Verification items for the finished model (mm, model axes). Face numbers are marked on the shaded views. A direction names the side the tool comes from. Round coordinates to 2 decimals unless told otherwise and drop trailing zeros. Write each loop counter-clockwise with the first axis right and the second up, starting at its lowest first coordinate (ties: lowest second). Pieces come first, ordered by that corner, then holes. Notation, with made-up numbers: M 49,-27.75 L 101,-27.75 A14 ccw 101,-20.75 Z; hole C 0.25,25.25 d8. An arc over 180 degrees is marked long. One line per question, with ' | ' between items.
Autodesk Inventor part; units mm, degrees
ref_plane "YZ Plane" through (0, 0, 0) normal (1, 0, 0) x (0, 1, 0)
ref_plane "XZ Plane" through (0, 0, 0) normal (0, 1, 0) x (-1, 0, 0)
ref_plane "XY Plane" through (0, 0, 0) normal (0, 0, 1) x (1, 0, 0)
sketch "Sketch4" plane through (0, 0, 0) normal (0, 0, 1) x (1, 0, 0)
  line L0 (-1.6, 0) -> (5, 0)
  line L1 (0, 0) -> (-1.6, 0)
  line L2 (0, 2) -> (0, 1.38)
  line L3 (0.4, 0.98) -> (0.4, 0.98)
  line L4 (0.4, 0.98) -> (0.8, 1)
  arc A0 (0, 1.38) -> (0.4, 0.98) centre (0.4, 1.38) ccw
  line L5 (-1.6, 0) -> (-1.6, 1)
  line L6 (0, 2) -> (-0.83, 2)
  arc A1 (-0.83, 2) -> (-1.6, 1) centre (1.2707, -0.414) ccw
  line L7 (0.8, 1) -> (5, 1)
  line L8 (5, 1) -> (5, 0)
  point P0 (0, 0.98)
  dimension "d71" = 0.4
  dimension "d72" = 5
  dimension "d74" = 0.4
  dimension "d75" = 1.96
  dimension "d78" = 2
  dimension "d82" = 3.2
  dimension "d83" = 1.6
  dimension "d84" = 4
  dimension "d104" = 4.2
  dimension "d105" = 2
revolve "Revolution7" add sketch "Sketch4" angle 360 about axis through (-1.6, 0, 0) along (1, 0, 0)
sketch "Sketch5" plane through (-1.6, 0, 0) normal (-1, 0, 0) x (0, 0, 1)
  circle A0 centre (0, 0) radius 0.875 construction
  circle A1 centre (0, 0) radius 0.6125 construction
  line L0 (0, 0) -> (-0.5304, 0.3062)
  line L1 (0, 0) -> (-0.5304, -0.3063)
  line L2 (-1.8008, 0) -> (1.7887, 0)
  line L3 (-0.875, 0) -> (-0.5304, -0.3063)
  line L4 (-0.875, 0) -> (-0.5304, 0.3062)
  point P0 (0, 0)
  dimension "d88" = 1.75
  dimension "d89" = 1.225
  dimension "d90" = 30
  dimension "d91" = 30
extrude "Extrusion1" cut sketch "Sketch5" against normal blind 0.77
pattern_circular "Circular Pattern1" count 6 over 360 about axis through (-10, 0, 0) along (1, 0, 0) of "Extrusion1"
fillet "Fillet1" radius 0.175 12 edges at (-1.215, -0.7578, -0.4375) (-1.215, -0.3063, -0.5304) (-1.215, -0.6125, 0) (-1.215, -0.7578, 0.4375) (-1.215, -0.3062, 0.5304) (-1.215, 0, 0.875) (-1.215, 0.6125, 0) (-1.215, 0.7578, 0.4375) (-1.215, 0.3063, 0.5304) (-1.215, 0.3062, -0.5304) (-1.215, 0, -0.875) (-1.215, 0.7578, -0.4375)
thread "Thread7"
properties part number "Šroub s válcovou hlavou a šestiramennou drážkou ISO 14583 - M2 x 5 - 4.8" material "Ocel, měkká"
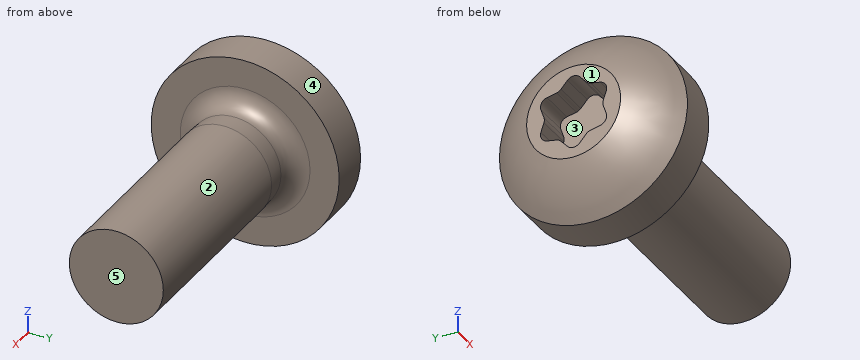
1. Go/stop test with a flat-tipped pin: P1, Ø2, axis at x = 3.5, z = 1, coming from the -Y side. Record where the tip stops, or that it passes through.
Results:
P1: stops at y = -1
2. Section check A-A, the plane x = 2.75. Record the cut outline in (y, z).
Results:
outline: C 0,0 d2
3. Mould release check, pull along Y, two halves, no side actions. Record for the marked faces 3, 4 and 5: pulls with the +Y half, pulls with the -Y half, needs draft (parallel to the pull), parting line crosses it, or undercut.
Results:
face 3: undercut | face 4: parting line crosses it | face 5: needs draft
4. Tool access check on the marked faces 1 and 2. Record the directions out of +Z, -Z, +X, -X, +Y, -Y that give a thin tool (end or side, any length) a straight path to the whole face; none if there is none.
Results:
face 1: +Z, -Z, -X, +Y, -Y | face 2: +X
5. Thickness scan on line 1 (Z direction, x = 2.5, y = 0.05); line 2 (Y direction, x = 1, z = 0.4); line 3 (X direction, y = 1.3, z = 1.35). Record the ranges inside material, lowest first.
Results:
line 1: z = -1 to 1 | line 2: y = -0.92 to 0.92 | line 3: x = -0.97 to 0
